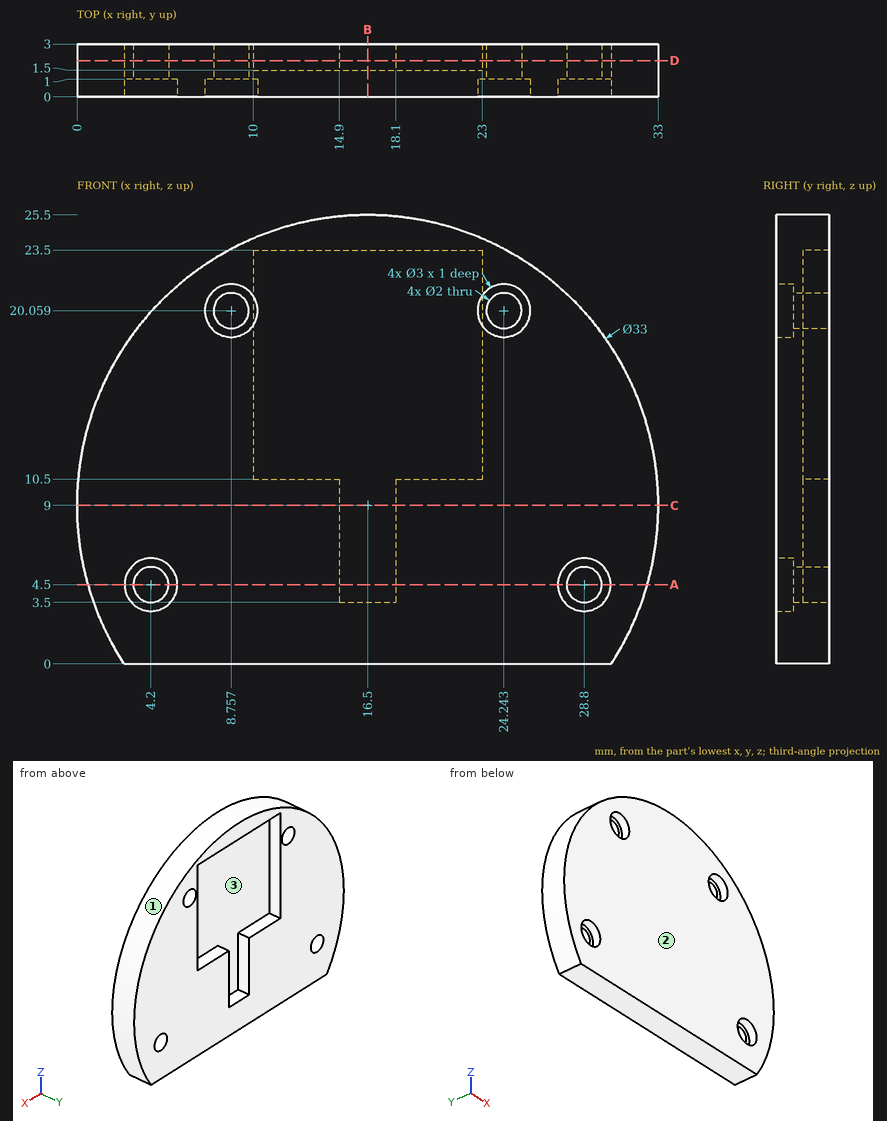
Study the drawing (mm; zero at the part's minimum x, y, z) and answer. Coordinates: 2 decimals unless noted, no trailing zeros. Write each loop counter-clockwise with the first axis right and the second up, starting at its lowest first coordinate (ties: lowest second). Pieces come first, ordered by that corner, then holes. Notation, with made-up numbers: (37.25, -18) - (44.25, -18) arc R19 ccw to (44.25, -9) - close; hole circle Ø3 at (7.25, 29). An arc over 180 degrees is marked (long way). Answer as a JSON object with one key per item and string values. Group by question number.
1. Each of these flat-tipped pins is pushed along its axis until it touches: P1, Ø1.2, axis at y = 2, z = 6, coming from the -X side (1 decimal); P2, Ø1.2, axis at y = 2.5, z = 16.5, coming from the -X side; P3, Ø1.6, axis at x = 12, y = 2, coming from the +Z side; P4, Ø3.5, axis at x = 24.24, z = 20.06, coming from the +Y side. Where does it stop, or does it pass through?
2. A cutting plane is placed at D-D (y = 2.05). Determine the outline of the cut face in (x, z), plus the area to 3 significant figures.
3. Consider L1, parallel to Y at x = 19, z = 19.5; L2, parallel to Y at x = 5, z = 5.25; L3, parallel to X at y = 1.65, z = 8.5. Determine where each line is inside the solid, lowest interval first. Write a range as [from, to].
4. The mould has two halves that part along X. Classify the marked faces 1, 2 and 3: +X half, -X half, draft (parallel to the pull), parting line (faces both ways), or undercut.
5. A cutting plane is placed at C-C (z = 9). Determine the outline of the cut face in (x, y).
6. A cutting plane is placed at B-B (x = 16.5). Determine the outline of the cut face in (y, z).
7. A cutting plane is placed at A-A (z = 4.5). Determine the outline of the cut face in (x, y) (1 decimal).
Worked out:
{
 "1": {"P1": "stops at x = 0.2", "P2": "stops at x = 1.51", "P3": "stops at z = 25.08", "P4": "stops at y = 3"},
 "2": {"outline": "(2.67, 0) - (30.33, 0) arc R16.5 ccw (long way) to start; hole circle Ø2 at (4.2, 4.5); hole circle Ø2 at (8.76, 20.06); hole (10, 10.5) - (14.9, 10.5) - (14.9, 3.5) - (18.1, 3.5) - (18.1, 10.5) - (23, 10.5) - (23, 23.5) - (10, 23.5) - close; hole circle Ø2 at (24.24, 20.06); hole circle Ø2 at (28.8, 4.5)", "area": "505 mm²"},
 "3": {"L1": "y = [0, 1.5]", "L2": "y = [1, 3]", "L3": "x = [0.01, 14.9], [18.1, 32.99]"},
 "4": {"face 1": "parting line", "face 2": "draft", "face 3": "undercut"},
 "5": {"outline": "(0, 0) - (33, 0) - (33, 3) - (18.1, 3) - (18.1, 1.5) - (14.9, 1.5) - (14.9, 3) - (0, 3) - close"},
 "6": {"outline": "(0, 0) - (3, 0) - (3, 3.5) - (1.5, 3.5) - (1.5, 23.5) - (3, 23.5) - (3, 25.5) - (0, 25.5) - close"},
 "7": {"outline": "(0.6, 0) - (2.7, 0) - (2.7, 1) - (3.2, 1) - (3.2, 3) - (0.6, 3) - close; (5.2, 1) - (5.7, 1) - (5.7, 0) - (27.3, 0) - (27.3, 1) - (27.8, 1) - (27.8, 3) - (18.1, 3) - (18.1, 1.5) - (14.9, 1.5) - (14.9, 3) - (5.2, 3) - close; (29.8, 1) - (30.3, 1) - (30.3, 0) - (32.4, 0) - (32.4, 3) - (29.8, 3) - close"}
}
